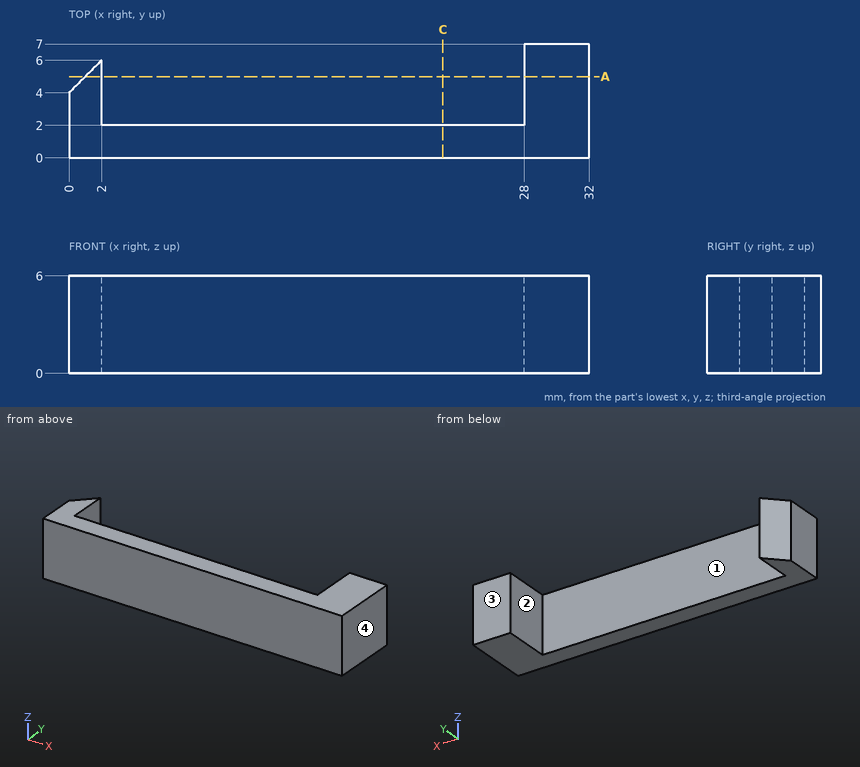
Can you work these out from the drawing? Everything is in mm from the part's minimum corner. Coordinates: 2 decimals unless noted, no trailing zeros. Order: outer loops, then holes, each group sorted by start corner. A loop starts at its lowest first (then second) coordinate and runs counter-clockwise, first axis right, second up. Notation, with made-up numbers: (71.25, 85) -> (112.25, 85) arc R20 ccw to (112.25, 104) -> close; hole circle Ø6 at (48.25, 38.5). An arc over 180 degrees is marked (long way). Return JSON: item names as keys, results as strings.
1) Thinking about a two-plate mould opening in X: for the marked faces 1, 2, 3 and 4, which applies, +X half, -X half, draft (parallel to the pull), parting line (faces both ways), or undercut?
Conclusion:
{"face 1": "undercut", "face 2": "undercut", "face 3": "draft", "face 4": "+X half"}
2) If I drill on probe 1 along X at (y, z) = (2.25, 5); probe 2 along X at (y, z) = (6.75, 1.5); probe 3 along Y at (x, z) = (27.5, 3), over which ranges is the centre line in solid material (lowest first)?
Conclusion:
{"probe 1": "x = 0 to 2, 28 to 32", "probe 2": "x = 28 to 32", "probe 3": "y = 0 to 2"}
3) If we section it at A-A on y = 5: List the corners of the cut face in (x, z) for me, plus the area to 3 significant figures.
Conclusion:
{"outline": "(1, 0) -> (2, 0) -> (2, 6) -> (1, 6) -> close; (28, 0) -> (32, 0) -> (32, 6) -> (28, 6) -> close", "area": "30.0 mm²"}
4) If we section it at C-C on x = 23: List the corners of the cut face in (y, z) for me, plus the area to 3 significant figures.
Conclusion:
{"outline": "(0, 0) -> (2, 0) -> (2, 6) -> (0, 6) -> close", "area": "12.0 mm²"}
5) I'm going to push a flat-ended pin straight in: P1, Ø2, axis at x = 4.5, y = 4.5, coming from the +Z side. Where does the tip first touch, or does it pass through?
Conclusion:
{"P1": "passes through"}
